Autodesk Inventor part; units mm, degrees
ref_plane "YZ Plane" through (0, 0, 0) normal (1, 0, 0) x (0, 1, 0)
ref_plane "XZ Plane" through (0, 0, 0) normal (0, 1, 0) x (-1, 0, 0)
ref_plane "XY Plane" through (0, 0, 0) normal (0, 0, 1) x (1, 0, 0)
sketch "Sketch1" plane through (0, 0, 0) normal (1, 0, 0) x (0, 1, 0)
  circle A0 centre (0, 0) radius 22.25
  circle A1 centre (0, 0) radius 8.625
  line L0 (8.625, 0) -> (22.25, 0) construction
  line L1 (21.91, 3.875) -> (7.7055, 3.875) construction
  line L2 (7.7055, -3.875) -> (21.91, -3.875) construction
  circle A2 centre (-14, 0) radius 3.0375
  circle A3 centre (-4.3262, -13.3148) radius 3.0375
  circle A4 centre (11.3262, -8.229) radius 3.0375
  circle A5 centre (11.3262, 8.229) radius 3.0375
  circle A6 centre (-4.3262, 13.3148) radius 3.0375
  dimension "d0" = 44.5
  dimension "d1" = 17.25
  dimension "d2" = 7.75
  dimension "d3" = 3.875
  dimension "d4" = 0
  dimension "d5" = 6.075
  dimension "d32" = 14
  dimension "d35" = 360
extrude "Extrusion1" add sketch "Sketch1" along normal blind 2
sketch "Sketch2" plane through (0, 0, 0) normal (-1, 0, 0) x (0, 0, 1)
  circle A0 centre (0, 0) radius 8.625
  circle A1 centre (0, 0) radius 22.25
extrude "Extrusion2" add sketch "Sketch2" along normal blind 0.25
sketch "Sketch3" plane through (2, 0, 0) normal (1, 0, 0) x (0, 0, -1)
  line L0 (-3.1, 26.8099) -> (3.1, 26.8099)
  line L1 (3.1, 26.8099) -> (3.1, 14.25)
  line L2 (3.1, 14.25) -> (-3.1, 14.25)
  line L3 (-3.1, 14.25) -> (-3.1, 26.8099)
  circle A0 centre (0, 0) radius 22.25 construction
  line L4 (-2.05, 26.8099) -> (2.05, 26.8099)
  line L5 (2.05, 26.8099) -> (2.05, 14.25)
  line L6 (2.05, 14.25) -> (-2.05, 14.25)
  line L7 (-2.05, 14.25) -> (-2.05, 26.8099)
  line L8 (-26.4557, 5.3365) -> (-24.5398, 11.233)
  line L9 (-24.5398, 11.233) -> (-12.5946, 7.3518)
  line L10 (-12.5946, 7.3518) -> (-14.5105, 1.4552)
  line L11 (-14.5105, 1.4552) -> (-26.4557, 5.3365)
  line L12 (-26.1313, 6.3351) -> (-24.8643, 10.2344)
  line L13 (-24.8643, 10.2344) -> (-12.9191, 6.3532)
  line L14 (-12.9191, 6.3532) -> (-14.186, 2.4538)
  line L15 (-14.186, 2.4538) -> (-26.1313, 6.3351)
  line L16 (-13.2505, -23.5118) -> (-18.2664, -19.8676)
  line L17 (-18.2664, -19.8676) -> (-10.8839, -9.7064)
  line L18 (-10.8839, -9.7064) -> (-5.868, -13.3506)
  line L19 (-5.868, -13.3506) -> (-13.2505, -23.5118)
  line L20 (-14.1, -22.8947) -> (-17.417, -20.4847)
  line L21 (-17.417, -20.4847) -> (-10.0344, -10.3235)
  line L22 (-10.0344, -10.3235) -> (-6.7175, -12.7335)
  line L23 (-6.7175, -12.7335) -> (-14.1, -22.8947)
  line L24 (18.2664, -19.8676) -> (13.2505, -23.5118)
  line L25 (13.2505, -23.5118) -> (5.868, -13.3506)
  line L26 (5.868, -13.3506) -> (10.8839, -9.7064)
  line L27 (10.8839, -9.7064) -> (18.2664, -19.8676)
  line L28 (17.417, -20.4847) -> (14.1, -22.8947)
  line L29 (14.1, -22.8947) -> (6.7175, -12.7335)
  line L30 (6.7175, -12.7335) -> (10.0344, -10.3235)
  line L31 (10.0344, -10.3235) -> (17.417, -20.4847)
  line L32 (24.5398, 11.233) -> (26.4557, 5.3365)
  line L33 (26.4557, 5.3365) -> (14.5105, 1.4552)
  line L34 (14.5105, 1.4552) -> (12.5946, 7.3518)
  line L35 (12.5946, 7.3518) -> (24.5398, 11.233)
  line L36 (24.8643, 10.2344) -> (26.1313, 6.3351)
  line L37 (26.1313, 6.3351) -> (14.186, 2.4538)
  line L38 (14.186, 2.4538) -> (12.9191, 6.3532)
  line L39 (12.9191, 6.3532) -> (24.8643, 10.2344)
  dimension "d15" = 6.2
  dimension "d16" = 3.1
  dimension "d17" = 8
  dimension "d22" = 0
  dimension "d23" = 0
  dimension "d24" = 1.05
  dimension "d25" = 1.05
  dimension "d28" = 360
extrude "Extrusion3" cut sketch "Sketch3" against normal up to surface (2.25 mm away)
equation "\"d3\" = 0.5 * d2"
equation "\"d25\" = d24"
properties part number "Magnetic Disk"
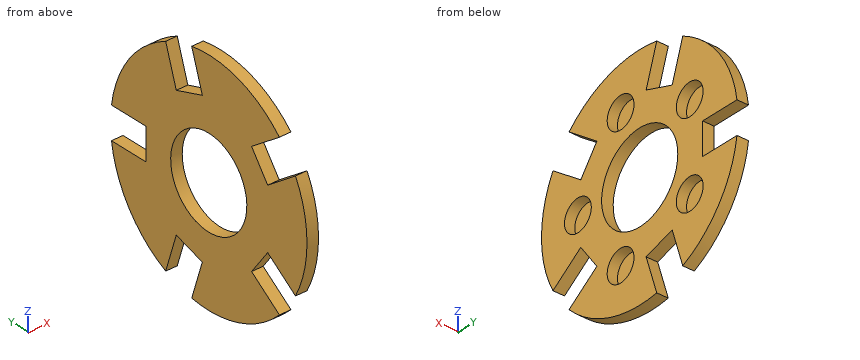
CAD build for the part. Positions are in the model's coordinates, mm. Round coordinates to 2 decimals unless told otherwise and drop trailing zeros. Order: outer loops, then holes, each group sorted by start corner. A loop starts at its lowest first (then second) coordinate and runs counter-clockwise, first axis right, second up. Notation, with made-up numbers: (3, -19.5) - (49, -19.5) arc R33 cw to (49, 17.5) - close; hole circle Ø8 at (-35.75, 84.25). An arc over 180 degrees is marked (long way). Return JSON: item names as keys, results as strings.
(1) Wall check: probe 1 along Z at (x, y) = (0.45, -13); probe 2 along Z at (x, y) = (0.75, 0) (3 decimals); probe 3 along Z at (x, y) = (1.2, -14). Give the ranges that are in metal, low to high. Write a range as from..to.
Answer key:
{"probe 1": "z = -18.06..-13.28, -6.35..-2.87, 2.87..6.35, 13.28..18.06", "probe 2": "z = -22.25..-8.625, 8.625..22.25", "probe 3": "z = -17.29..-14, -6.34..-3.04, 3.04..6.34, 14..17.29"}
(2) Cut at D-D (y = 16.5). Give the cut face in (x, z), then the cut area to 3 significant figures.
Answer key:
{"outline": "(-0.25, -14.93) - (2, -14.93) - (2, -3.1) - (-0.25, -3.1) - close; (-0.25, 3.1) - (2, 3.1) - (2, 14.93) - (-0.25, 14.93) - close", "area": "53.2 mm^2"}
(3) Pin check, flat tips, straight feed: pin 1 Ø0.7 at (x, y) = (0.5, 16.5) entering from -Z; pin 2 Ø12 at (y, z) = (1.5, 2) entering from -X; pin 3 Ø1.8 at (y, z) = (-15, 0.5) entering from +X. Stop position of each tip, or through.
Answer key:
{"pin 1": "stops at z = -15.3", "pin 2": "passes through", "pin 3": "stops at x = 0"}
(4) Cut at B-B (z = -4.5). Give the cut face in (x, y).
Answer key:
{"outline": "(-0.25, -21.79) - (2, -21.79) - (2, -7.36) - (-0.25, -7.36) - close; (-0.25, 7.36) - (2, 7.36) - (2, 21.79) - (-0.25, 21.79) - close"}
(5) Cut at C-C (x = 0.55). State how many separate pieces and enclosed holes the cut face has, then the cut area to 3 significant figures.
Answer key:
{"separate pieces": "1", "enclosed holes": "6", "area": "931 mm^2"}
(6) Cut at A-A (y = -14). Give the cut face in (x, z).
Answer key:
{"outline": "(-0.25, -17.29) - (2, -17.29) - (2, -14) - (-0.25, -14) - close; (-0.25, -6.34) - (2, -6.34) - (2, -3.04) - (0, -3.04) - (0, 3.04) - (2, 3.04) - (2, 6.34) - (-0.25, 6.34) - close; (-0.25, 14) - (2, 14) - (2, 17.29) - (-0.25, 17.29) - close"}
